Geometry: final body of the model. Coordinates: model frame, mm. A direction names the side the tool comes from. Give positions to 0.01 mm unless a question says otherwise; leave off trailing zeros. Write each loop counter-clockwise with the first axis right and the second up, starting at its lowest first coordinate (ties: lowest second). Pieces come first, ordered by that corner, then holes. Notation, with made-up numbers: (82, 34) -> (98, 34) arc R23 ccw to (98, 57) -> close; hole circle Ø11 at (59, -3.75). An arc over 180 degrees is marked (long way). Answer as a JSON object with one key per item and string values.
from build123d import *

# Parameters (mm, degrees)
SKETCH1_R               = 2.1828125
BOSS_EXTRUDE1_DEPTH     = 9.525
CUT_EXTRUDE2_DEPTH      = 4.365625
CUT_EXTRUDE3_DEPTH      = 109.557926934
CUT_EXTRUDE3_DEPTH_BACK = 109.557926934
SKETCH6_R               = 2.1828125
CHAMFER1_SIZE           = 0.396875


with BuildPart() as part:
    # Sketch1 → Boss-Extrude1 (new body)
    with BuildSketch(Plane(origin=(0, 0, 0), x_dir=(1, 0, 0), z_dir=(0, 1, 0))):
        with BuildLine():
            Line((0, -4.7625), (-1.859871939, -4.7625))
            ThreePointArc((-1.859871939, -4.7625), (-3.074891837, -5.004182484), (-4.10493597, -5.69243597))
            Line((-4.10493597, -5.69243597), (-18.182789755, -19.770289755))
            ThreePointArc((-18.182789755, -19.770289755), (-18.736403184, -19.880410313), (-19.05, -19.41107951))
            Line((-19.05, -19.41107951), (-19.05, -5.55625))
            ThreePointArc((-19.05, -5.55625), (-19.282483992, -4.994983992), (-19.84375, -4.7625))
            Line((-19.84375, -4.7625), (-101.6, -4.7625))
            ThreePointArc((-101.6, -4.7625), (-106.3625, 0), (-101.6, 4.7625))
            Line((-101.6, 4.7625), (0, 4.7625))
            ThreePointArc((0, 4.7625), (4.7625, 0), (0, -4.7625))
        make_face()
        with Locations(Location((0, 0, 0), (0, 0, 90))):
            Circle(SKETCH1_R, mode=Mode.SUBTRACT)
        with Locations(Location((-50.8, 0, 0), (0, 0, 90))):
            Circle(SKETCH1_R, mode=Mode.SUBTRACT)
        with Locations(Location((-101.6, 0, 0), (0, 0, 90))):
            Circle(SKETCH1_R, mode=Mode.SUBTRACT)
    extrude(amount=BOSS_EXTRUDE1_DEPTH)

    # Sketch5 → Cut-Extrude2 (cut)
    with BuildSketch(Plane.XY.offset(4.7625)):
        Polygon((-20.359010462, 4.7625), (-22.879505231, 9.128125), (-27.920494769, 9.128125), (-30.440989538, 4.7625), (-27.920494769, 0.396875), (-22.879505231, 0.396875), align=None)
        Polygon((-33.059010462, 4.7625), (-35.579505231, 9.128125), (-40.620494769, 9.128125), (-43.140989538, 4.7625), (-40.620494769, 0.396875), (-35.579505231, 0.396875), align=None)
    extrude(amount=-CUT_EXTRUDE2_DEPTH, mode=Mode.SUBTRACT)

    # Sketch6 → Cut-Extrude3 (cut, two sides: drawn at the far end of the back side and taken through both)
    with BuildSketch(Plane.XY.offset(0.396875).offset(-CUT_EXTRUDE3_DEPTH_BACK)):
        with Locations((-38.1, 4.7625)):
            Circle(SKETCH6_R)
        with Locations((-25.4, 4.7625)):
            Circle(SKETCH6_R)
    extrude(amount=CUT_EXTRUDE3_DEPTH + CUT_EXTRUDE3_DEPTH_BACK, mode=Mode.SUBTRACT)

    # Chamfer1
    chamfer1_edges = [part.edges().sort_by_distance(p)[0] for p in [
        (-0.92993597, 0, 4.7625),
        (-3.074891837, 0, 5.004182484),
        (-11.143862862, 0, 12.731362862),
        (-18.736403184, 0, 19.880410313),
        (-19.05, 0, 12.483664755),
        (-19.282483992, 0, 4.994983992),
        (-60.721875, 0, 4.7625),
        (-106.3625, 9.525, 0),
        (-106.3625, 0, 0),
        (-50.8, 0, -4.7625),
        (4.7625, 0, 0),
        (-60.721875, 9.525, 4.7625),
        (-19.282483992, 9.525, 4.994983992),
        (-19.05, 9.525, 12.483664755),
        (0, 0, 2.1828125),
        (0, 9.525, 2.1828125),
        (-18.736403184, 9.525, 19.880410313),
        (-50.8, 0, 2.1828125),
        (-50.8, 9.525, 2.1828125),
        (-11.143862862, 9.525, 12.731362862),
        (-101.6, 0, 2.1828125),
        (-101.6, 9.525, 2.1828125),
        (-3.074891837, 9.525, 5.004182484),
        (-0.92993597, 9.525, 4.7625),
        (4.7625, 9.525, 0),
        (-40.2828125, 4.7625, 0.396875),
        (-40.2828125, 4.7625, -4.7625),
        (-27.5828125, 4.7625, 0.396875),
        (-27.5828125, 4.7625, -4.7625),
        (-50.8, 9.525, -4.7625),
    ]]
    chamfer(chamfer1_edges, length=CHAMFER1_SIZE - 0.0001)  # a hair under: the kernel refuses the full size


solid = part.part
Q1. Mould query, pull axis Z, two halves, no side actions, for faces 1 (the cylindrical face through (-52.964, 4.701, 0.284)), 2 (the conical face through (-106.072, 0.107, 0.098)), 3 (the flat face through (-21.6, 6.91, 2.61)). Classes: pulls with the +Z half, pulls with the -Z half, needs draft (parallel to the pull), parting line crosses it, or undercut.
Values:
{"face 1": "undercut", "face 2": "parting line crosses it", "face 3": "needs draft"}
Q2. Set-up query: faces 4 (the flat face through (-1, 5, 4.762)), 5 (the flat face through (-34.337, 2.549, 2.61)), 6 (the flat face through (-46, 0, 2)). Return all of +Z, -Z, +X, -X, +Y, -Y with unobstructed straight access to the full face (end or side cutting, diameter ignored); none if empty.
Values:
{"face 4": "+Z, +X, +Y, -Y", "face 5": "+Z", "face 6": "+Z, -Z, +X, -X, -Y"}
Q3. Cut plane D-D (y = 5.75). State how many separate pieces and enclosed holes the cut face has, and give its area (3 significant figures).
Values:
{"separate pieces": "3", "enclosed holes": "3", "area": "1,000 mm²"}
Q4. First-contact query: P1, Ø5, axis at y = 4.5, z = 16, coming from the -X side; P2, Ø1.5, axis at x = -21, y = 3.5, coming from the +Z side; P3, Ø4.5, axis at x = -38, y = 6, coming from the +Z side. Flat tips, straight axial feed; report the tip coordinate or a pass-through.
Values:
{"P1": "x = -19.05", "P2": "z = 4.76", "P3": "z = 0.4"}
Q5. Cut plane C-C (x = -50.8). Return the cut outline in (y, z) (1 decimal).
Values:
{"outline": "(0, -4.4) -> (0.4, -4.8) -> (9.1, -4.8) -> (9.5, -4.4) -> (9.5, -2.6) -> (9.1, -2.2) -> (0.4, -2.2) -> (0, -2.6) -> close; (0, 2.6) -> (0.4, 2.2) -> (9.1, 2.2) -> (9.5, 2.6) -> (9.5, 4.4) -> (9.1, 4.8) -> (0.4, 4.8) -> (0, 4.4) -> close"}
Q6. Material intervals for L1, parallel to X at y = 4.5, z = 0; L2, parallel to Y at x = -25.4, z = -2.8 (3 decimals); L3, parallel to X at y = 8.75, z = 3.25, sorted ascending. Write a range as from..to.
Values:
{"L1": "-106.36..-103.78, -99.42..-52.98, -48.62..-40.27, -35.93..-27.57, -23.23..-2.18, 2.18..4.76", "L2": "0..2.58, 6.945..9.525", "L3": "-105.08..-40.84, -35.36..-28.14, -22.66..3.48"}
